Autodesk Inventor part; units mm, degrees
ref_plane "YZ Plane" through (0, 0, 0) normal (1, 0, 0) x (0, 1, 0)
ref_plane "XZ Plane" through (0, 0, 0) normal (0, 1, 0) x (-1, 0, 0)
ref_plane "XY Plane" through (0, 0, 0) normal (0, 0, 1) x (1, 0, 0)
sketch "스케치1" plane through (0, 0, 0) normal (0, 1, 0) x (-1, 0, 0)
  line L0 (-12, 27) -> (12, 27)
  line L1 (12, 27) -> (12, -27)
  line L2 (12, -27) -> (-12, -27)
  line L3 (-12, -27) -> (-12, 27)
  line L4 (-12, 27) -> (12, -27) construction
  line L5 (12, 27) -> (-12, -27) construction
  circle A0 centre (9.5, 18) radius 1.5
  circle A1 centre (-9.7, -17) radius 1.5
  point P0 (0, 0)
  dimension "d0" = 24
  dimension "d1" = 54
  dimension "d2" = 3
  dimension "d3" = 9
  dimension "d4" = 2.5
  dimension "d5" = 3
  dimension "d6" = 10
  dimension "d7" = 2.3
extrude "돌출1" add sketch "스케치1" along normal blind 1.5
sketch "스케치2" plane through (0, 1.5, 0) normal (0, 1, 0) x (1, 0, 0)
  circle A0 centre (0, -21.5) radius 5
  circle A1 centre (0, 21.5) radius 5
  line L0 (12, 27) -> (-12, 27)
  line L1 (-12, -27) -> (12, -27)
  point P0 (0, 0)
  dimension "d10" = 10
  dimension "d11" = 5.5
  dimension "d12" = 5.5
  dimension "d13" = 10
extrude "돌출2" add sketch "스케치2" along normal blind 10.5
sketch "스케치3" plane through (0, 1.5, 0) normal (0, 1, 0) x (1, 0, 0)
  line L0 (-6.5682, -3.4773) -> (3.2197, -3.4773)
  line L1 (3.2197, -3.4773) -> (3.2197, 13.5227)
  line L2 (3.2197, 13.5227) -> (-6.5682, 13.5227)
  line L3 (-6.5682, 13.5227) -> (-6.5682, -3.4773)
  line L4 (-6.5682, -3.4773) -> (3.2197, 13.5227) construction
  line L5 (3.2197, -3.4773) -> (-6.5682, 13.5227) construction
  point P0 (0, 0)
  point P1 (-1.6742, 5.0227)
  dimension "d16" = 17
extrude "돌출3" add sketch "스케치3" along normal blind 14.5
properties part number "스텝다운 컨버터"
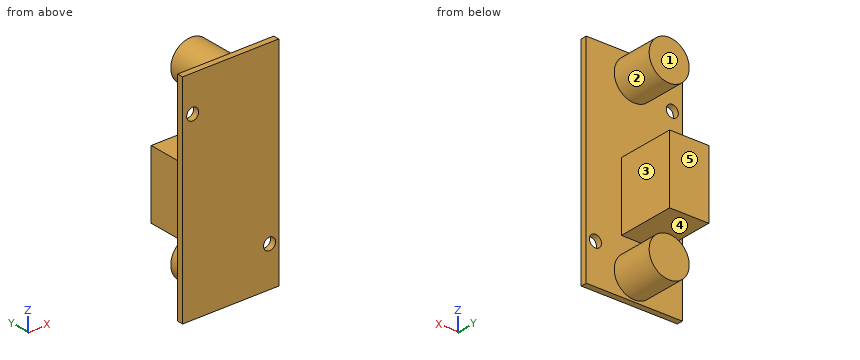
Could you check a few things on this model? Use its own coordinates, in mm. Face numbers are marked on the shaded views. A direction names the side the tool comes from. Round coordinates to 2 decimals unless told otherwise and drop trailing zeros. Loops run counter-clockwise (first coordinate to the right, second up) from the corner with the lowest first, then second, coordinate; pieces in that order, holes last. Notation, with made-up numbers: (52.25, 72.25) -> (77.25, 72.25) arc R28 ccw to (77.25, 100.25) -> close; hole circle Ø2 at (-2, 5.5). An arc over 180 degrees is marked (long way). One line per question, with ' | ' between items.
(1) If I drill on probe 1 along Z at (x, y) = (-9.5, 0.9); probe 2 along Z at (x, y) = (9.7, 1); probe 3 along Z at (x, y) = (-1.5, 8.5), over which ranges is the centre line in solid material (lowest first)?
Model answer:
probe 1: z = -27 to 16.5, 19.5 to 27 | probe 2: z = -27 to -18.5, -15.5 to 27 | probe 3: z = -26.27 to -16.73, -13.52 to 3.48, 16.73 to 26.27
(2) If we section it at C-C on z = 17: List the corners of the cut face in (x, y) for me.
Model answer:
outline: (-12, 0) -> (-10.62, 0) -> (-10.62, 1.5) -> (-12, 1.5) -> close; (-8.38, 0) -> (12, 0) -> (12, 1.5) -> (2.18, 1.5) -> (2.18, 12) -> (-2.18, 12) -> (-2.18, 1.5) -> (-8.38, 1.5) -> close
(3) For the marked faces 1, 2 and 3, which set-ups out of +Z, -Z, +X, -X, +Y, -Y let a thin tool reach every point of the face, with its end or its side?
Model answer:
face 1: +Z, +X, -X, +Y | face 2: +Y | face 3: +X, +Y
(4) For pin 1 Ø5 at (x, z) = (1.5, -20.5) entering from +Y; pin 2 Ø2.5 at (x, z) = (9.7, -17) entering from +Y (3 decimals); pin 3 Ø5 at (y, z) = (11, 19.5) entering from +X; pin 4 Ø3 at (x, y) = (-1.5, 7) entering from +Z, each with a flat end and sliding along its axis, tell me the tip position at first contact or that it passes through.
Model answer:
pin 1: stops at y = 12 | pin 2: passes through | pin 3: stops at x = 5 | pin 4: stops at z = 26.5
(5) Thinking about a two-plate mould opening in Z: for the marked faces 4 and 5, which applies, released by +Z, released by -Z, zero draft, split by the parting line, or undercut?
Model answer:
face 4: undercut | face 5: zero draft
(6) If we section it at B-B on y = 7.25: List the corners of the cut face in (x, z) for me.
Model answer:
outline: (-6.57, -13.52) -> (3.22, -13.52) -> (3.22, 3.48) -> (-6.57, 3.48) -> close; circle Ø10 at (0, -21.5); circle Ø10 at (0, 21.5)
(7) If we section it at D-D on x = 0: List the corners of the cut face in (y, z) for me.
Model answer:
outline: (0, -27) -> (1.5, -27) -> (1.5, -26.5) -> (12, -26.5) -> (12, -16.5) -> (1.5, -16.5) -> (1.5, -13.52) -> (16, -13.52) -> (16, 3.48) -> (1.5, 3.48) -> (1.5, 16.5) -> (12, 16.5) -> (12, 26.5) -> (1.5, 26.5) -> (1.5, 27) -> (0, 27) -> close
(8) If we section it at A-A on x = -9.5: List the corners of the cut face in (y, z) for me.
Model answer:
outline: (0, -27) -> (1.5, -27) -> (1.5, 16.5) -> (0, 16.5) -> close; (0, 19.5) -> (1.5, 19.5) -> (1.5, 27) -> (0, 27) -> close
